Part print with two shaded views. Sizes in mm from the minimum x, y, z corner. Round coordinates to 2 decimals unless told otherwise and drop trailing zeros. Order: outer loops, then holes, each group sorted by start corner. A loop starts at its lowest first (then second) coordinate and runs counter-clockwise, first axis right, second up. Notation, with made-up numbers: M -18,88.25 L 11,88.25 A10 cw 11,101.25 Z; hole C 85,86.5 d8. An arc over 180 degrees is marked long. Put each result on its own line as item: value.
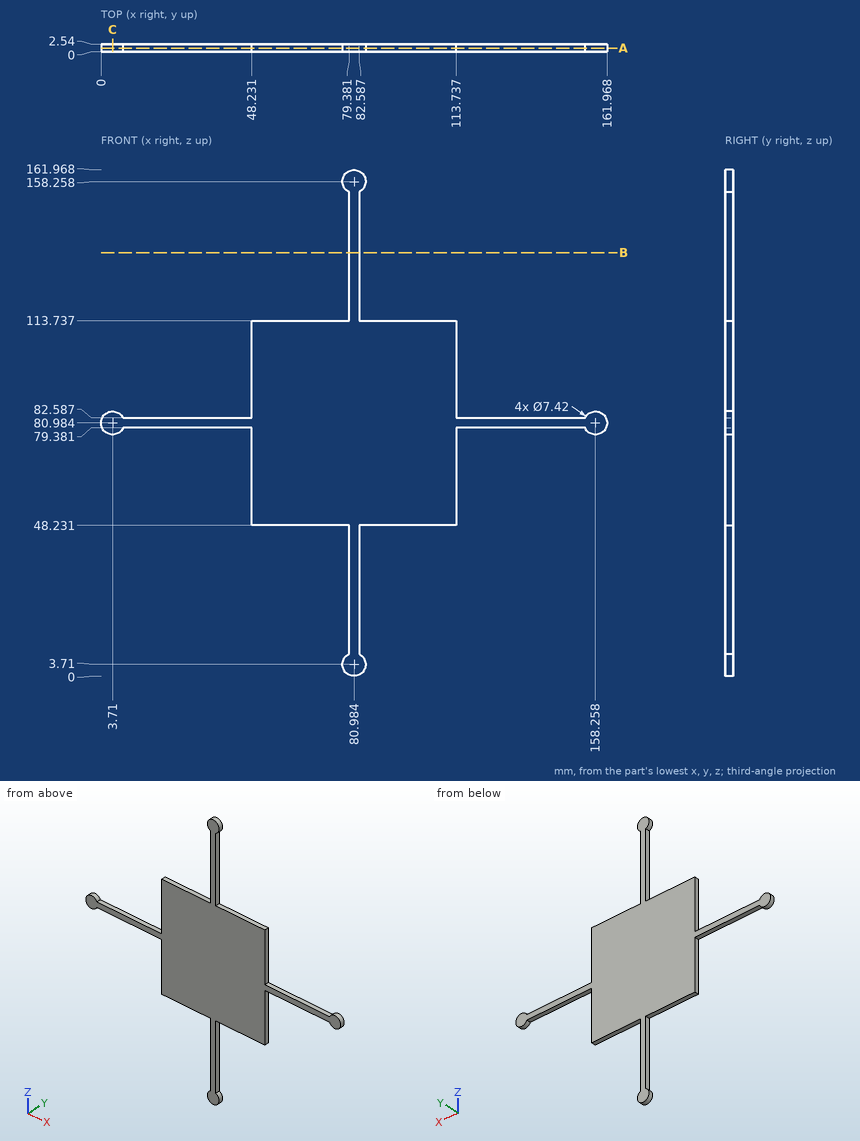
Item 1: Probe line 1 along Z through (x, y) = (78, 1.7) (1 decimal); line 2 along X through (y, z) = (1.55, 83) (1 decimal); line 3 along X through (y, z) = (2.1, 8). List the from-to ranges inside material, lowest first. Write a range as [from, to].
Answers below:
line 1: [1.5, 5.9], [48.2, 113.7], [156.1, 160.5]
line 2: [0.6, 6.8], [48.2, 113.7], [155.1, 161.4]
line 3: [79.38, 82.59]
Item 2: Band-saw the part on B-B on z = 135.5. Give the cut face in (x, y).
Answers below:
outline: M 79.38,0 L 82.59,0 L 82.59,2.54 L 79.38,2.54 Z
Item 3: Band-saw the part on C-C on x = 3.71. Give the cut face in (y, z).
Answers below:
outline: M 0,77.27 L 2.54,77.27 L 2.54,84.69 L 0,84.69 Z
Item 4: Pin check, flat tips, straight feed: P1, Ø1.3, axis at y = 1.5, z = 28, coming from the +X side; P2, Ø1.5, axis at y = 2.5, z = 40, coming from the -X side; P3, Ø1.3, axis at x = 131, y = 0.5, coming from the -Z side. Stop position of each tip, or through.
Answers below:
P1: x = 82.59
P2: x = 79.38
P3: z = 79.38
Item 5: Band-saw the part on A-A on y = 1.25. Give the cut face in (x, z).
Answers below:
outline: M 7.06,79.38 L 48.23,79.38 L 48.23,48.23 L 79.38,48.23 L 79.38,7.06 A3.71 ccw long 82.59,7.06 L 82.59,48.23 L 113.74,48.23 L 113.74,79.38 L 154.91,79.38 A3.71 ccw long 154.91,82.59 L 113.74,82.59 L 113.74,113.74 L 82.59,113.74 L 82.59,154.91 A3.71 ccw long 79.38,154.91 L 79.38,113.74 L 48.23,113.74 L 48.23,82.59 L 7.06,82.59 A3.71 ccw long Z
